Work out the finished part from the listing and answer in its coordinate system (mm). A direction names the side the tool comes from. Round coordinates to 2 decimals unless told otherwise and drop trailing zeros. Loops run counter-clockwise (first coordinate to the right, second up) from the corner with the lowest first, then second, coordinate; pieces in that order, holes last. Notation, with made-up numbers: (76, 55) -> (131, 55) arc R21 ccw to (131, 94) -> close; hole circle Ø11 at (-23.75, 55). An arc over 180 degrees is marked (long way). Use one line per item in the form item = value.
```python
from build123d import *

# Parameters (mm, degrees)
SKETCH1_W           = 20
SKETCH1_H           = 16
BOSS_EXTRUDE1_DEPTH = 14.5
CUT_EXTRUDE1_REACH  = 22
SKETCH2_W           = 13.1
SKETCH2_H           = 13.1


with BuildPart() as part:
    # Sketch1 → Boss-Extrude1 (new body)
    with BuildSketch(Plane(origin=(0, 0, 0), x_dir=(1, 0, 0), z_dir=(0, 1, 0))):
        Rectangle(SKETCH1_W, SKETCH1_H)
    extrude(amount=BOSS_EXTRUDE1_DEPTH)

    # Sketch2 → Cut-Extrude1 (cut, up to next)
    with BuildSketch(Plane.ZY.offset(10), mode=Mode.PRIVATE) as cut_extrude1_sk1:
        with Locations((0, 6.55)):
            Rectangle(SKETCH2_W, SKETCH2_H)
    cut_extrude1_tool1 = extrude(cut_extrude1_sk1.sketch, amount=-CUT_EXTRUDE1_REACH, mode=Mode.PRIVATE) & part.part
    add(cut_extrude1_tool1.solids().sort_by_distance((-10, 6.55, 0))[0], mode=Mode.SUBTRACT)


solid = part.part
```
(1) Find section A-A, the plane y = 7.25. Write down the section's boundary in (x, z).
Completed:
outline = (-10, -8) -> (10, -8) -> (10, -6.55) -> (-10, -6.55) -> close; (-10, 6.55) -> (10, 6.55) -> (10, 8) -> (-10, 8) -> close
(2) For a pull along Z with two mould halves and no side action, classify faces 1 (the flat face through (0, 7, 8)), 2 (the flat face through (0, 6, -6.55)), 3 (the flat face through (0, 0, 7)) as +Z half, -Z half, draft (parallel to the pull), parting line (faces both ways), or undercut.
Completed:
face_1 = +Z half
face_2 = undercut
face_3 = draft
(3) For faces 4 (the flat face through (0, 7, -8)), 5 (the flat face through (0, 13.1, 0)), determine the directions among +Z, -Z, +X, -X, +Y, -Y from which every point of the face is accessible in a straight line to the end or side of a thin tool.
Completed:
face_4 = -Z, +X, -X, +Y, -Y
face_5 = +X, -X, -Y
(4) Find section C-C, the plane z = 0.75. Write down the section's boundary in (x, y), then the cut area to 3 significant figures.
Completed:
outline = (-10, 13.1) -> (10, 13.1) -> (10, 14.5) -> (-10, 14.5) -> close
area = 28.0 mm2
(5) Given P1, Ø5, axis at y = 4.5, z = 3, coming from the -X side; P2, Ø2, axis at x = 6.5, z = 0, coming from the -Y side, each flat-ended and moving along its own axis, determine where each tip first touches the part or whether it passes through.
Completed:
P1 = through
P2 = 13.1
(6) Consider L1, parallel to Z at x = 4.75, y = 5; L2, parallel to Y at x = -9, z = -5. Determine where each line is inside the solid, lowest interval first.
Completed:
L1 = -8 to -6.55, 6.55 to 8
L2 = 13.1 to 14.5
(7) Find section B-B, the plane x = 1. Write down the section's boundary in (y, z), then the cut area to 3 significant figures.
Completed:
outline = (0, -8) -> (14.5, -8) -> (14.5, 8) -> (0, 8) -> (0, 6.55) -> (13.1, 6.55) -> (13.1, -6.55) -> (0, -6.55) -> close
area = 60.4 mm2
